For this review, take the finished solid that the model builds, in its own axes (mm). Face numbers are marked on the shaded views. A direction names the side the tool comes from. Round coordinates to 2 decimals unless told otherwise and drop trailing zeros. Loops run counter-clockwise (first coordinate to the right, second up) from the corner with the lowest first, then second, coordinate; pieces in that order, holes last.
1. To check wall thickness, follow line 1 along Z through (x, y) = (-94, 13); line 2 along Y through (x, z) = (-140, -29); line 3 along Z through (x, y) = (-28.5, 2). State the ranges of each line that lie inside material, in increasing order.
2. Clearance check with flat-ended pins moving along their axes: pin 1 Ø6 at (y, z) = (8.5, -155.5) entering from -X; pin 2 Ø3 at (x, z) = (-102.5, -101.5) entering from +Y. State where each tip first meets the part, or that it passes through.
3. Consider section B-B on x = -130.5. State the section outline as (y, z) points.
4. Consider section A-A on y = 36. State the section outline as (x, z) points.
5. Tool access review of the marked faces 1 and 2: name each direction out of +Z, -Z, +X, -X, +Y, -Y from which nothing blocks a thin tool from reaching the whole face with its end or side.
6. Consider section C-C on z = -184.5. State the section outline as (x, y) points.
Autodesk Inventor part; units mm, degrees
ref_plane "YZ Plane" through (0, 0, 0) normal (1, 0, 0) x (0, 1, 0)
ref_plane "XZ Plane" through (0, 0, 0) normal (0, 1, 0) x (-1, 0, 0)
ref_plane "XY Plane" through (0, 0, 0) normal (0, 0, 1) x (1, 0, 0)
sketch "Sketch1" plane through (0, 0, 0) normal (0, 1, 0) x (-1, 0, 0)
  line L0 (0, 0) -> (150, 0)
  line L1 (150, 0) -> (150, -200)
  line L2 (150, -200) -> (0, -200)
  line L3 (0, -200) -> (0, 0)
  dimension "d0" = 200
  dimension "d1" = 150
extrude "Plate1" add sketch "Sketch1" along normal blind 3
sketch "Sketch2" plane through (0, 0, -3) normal (0, 0, 1) x (1, 0, 0)
  line L0 (-150, 0) -> (0, 0)
  line L1 (0, 0) -> (0, 40)
  line L2 (0, 40) -> (-150, 40)
  line L3 (-150, 40) -> (-150, 0)
edge flange "Flange1" height 40 angle 90 thickness 3 bend radius 3 thickness toward (0, 0, 1) relief tear relief width 3 relief depth 1.5 edges at (-75, 3, 0) wall of the first edge with corners at (-150, 0, -3) (0, 0, -3) (0, 40, -3) (-150, 40, -3)
bend "Bend1"
corner "Corner1"
sketch "Sketch3" plane through (-150, 0, -197) normal (0, 0, -1) x (-1, 0, 0)
  line L0 (-150, 0) -> (0, 0)
  line L1 (0, 0) -> (0, 40)
  line L2 (0, 40) -> (-150, 40)
  line L3 (-150, 40) -> (-150, 0)
edge flange "Flange2" height 40 angle 90 thickness 3 bend radius 3 thickness toward (0, 0, -1) relief tear relief width 3 relief depth 1.5 edges at (-75, 3, -200) wall of the first edge with corners at (0, 0, -197) (-150, 0, -197) (-150, 40, -197) (0, 40, -197)
bend "Bend2"
corner "Corner2"
equation "\"d2\" = Thickness"
equation "\"d3\" = BendReliefWidth"
equation "\"d4\" = BendReliefDepth"
equation "\"d5\" = MinimumRemnant"
equation "\"d6\" = TransitionRadius"
equation "\"d9\" = BendRadius"
equation "\"d10\" = CornerReliefSize"
equation "\"d11\" = GapSize"
equation "\"d12\" = JacobiRadiusSize"
equation "\"d13\" = BendReliefWidth"
equation "\"d14\" = BendReliefDepth"
equation "\"d15\" = MinimumRemnant"
equation "\"d16\" = TransitionRadius"
equation "\"d19\" = BendRadius"
equation "\"d20\" = CornerReliefSize"
equation "\"d21\" = GapSize"
equation "\"d22\" = JacobiRadiusSize"
equation "\"BendRadius\" = Thickness"
equation "\"BendReliefWidth\" = Thickness"
equation "\"BendReliefDepth\" = 0.5 * Thickness"
equation "\"CornerReliefSize\" = 4 * Thickness"
equation "\"MinimumRemnant\" = 2 * Thickness"
equation "\"TransitionRadius\" = BendRadius"
equation "\"JacobiRadiusSize\" = BendRadius"
equation "\"GapSize\" = Thickness"
properties part number "floor" material "Aluminum 6061"
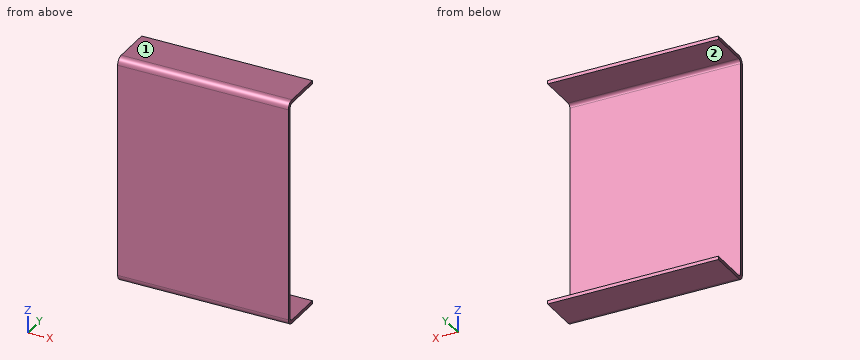
Resolved:
1. line 1: z = -200 to -197, -3 to 0
1. line 2: y = 0 to 3
1. line 3: z = -198.47 to -1.53
2. pin 1: passes through
2. pin 2: stops at y = 3
3. outline: (0, -194) arc R6 ccw to (6, -200) - (40, -200) - (40, -197) - (6, -197) arc R3 cw to (3, -194) - (3, -6) arc R3 cw to (6, -3) - (40, -3) - (40, 0) - (6, 0) arc R6 ccw to (0, -6) - close
4. outline: (-150, -200) - (0, -200) - (0, -197) - (-150, -197) - close; (-150, -3) - (0, -3) - (0, 0) - (-150, 0) - close
5. face 1: +Z, +X, -X, +Y, -Y
5. face 2: +X, -X, +Y
6. outline: (-150, 0) - (0, 0) - (0, 3) - (-150, 3) - close
